from build123d import *

# Parameters (mm, degrees)
BOSS_EXTRUDE1_DEPTH = 12
SKETCH3_R           = 11
CUT_EXTRUDE1_DEPTH  = 12
FILLET1_R           = 15
FILLET2_R           = 15
FILLET3_R           = 2
FILLET4_R           = 2
SKETCH4_R           = 2.5
CUT_EXTRUDE2_DEPTH  = 12
FILLET5_R           = 2
FILLET6_R           = 2
FILLET7_R           = 2
FILLET8_R           = 2


with BuildPart() as part:
    # Sketch2 → Boss-Extrude1 (new body)
    with BuildSketch(Plane(origin=(0, 0, 0), x_dir=(1, 0, 0), z_dir=(0, 1, 0))):
        Polygon((0, 0), (55, 0), (55, 5), (43, 5), (43, 30), (12, 30), (12, 5), (0, 5), align=None)
    extrude(amount=BOSS_EXTRUDE1_DEPTH)

    # Sketch3 → Cut-Extrude1 (cut)
    with BuildSketch(Plane.XZ):
        with Locations(Location((27.5, -17.5, 0), (0, 0, 270))):
            Circle(SKETCH3_R)
    extrude(amount=-CUT_EXTRUDE1_DEPTH, mode=Mode.SUBTRACT)

    # Fillet1
    fillet1_edges = [part.edges().sort_by_distance(p)[0] for p in [
        (43, 6, -30),
    ]]
    fillet(fillet1_edges, radius=FILLET1_R)

    # Fillet2
    fillet2_edges = [part.edges().sort_by_distance(p)[0] for p in [
        (12, 6, -30),
    ]]
    fillet(fillet2_edges, radius=FILLET2_R)

    # Fillet3
    fillet3_edges = [part.edges().sort_by_distance(p)[0] for p in [
        (12, 6, -5),
    ]]
    fillet(fillet3_edges, radius=FILLET3_R)

    # Fillet4
    fillet4_edges = [part.edges().sort_by_distance(p)[0] for p in [
        (43, 6, -5),
    ]]
    fillet(fillet4_edges, radius=FILLET4_R)

    # Sketch4 → Cut-Extrude2 (cut)
    with BuildSketch(Plane.XY):
        with Locations((48.5, 6.034122725)):
            Circle(SKETCH4_R)
        with Locations((6.5, 6.034122725)):
            Circle(SKETCH4_R)
    extrude(amount=-CUT_EXTRUDE2_DEPTH, mode=Mode.SUBTRACT)

    # Fillet5
    fillet5_edges = [part.edges().sort_by_distance(p)[0] for p in [
        (55, 0, -2.5),
    ]]
    fillet(fillet5_edges, radius=FILLET5_R)

    # Fillet6
    fillet6_edges = [part.edges().sort_by_distance(p)[0] for p in [
        (55, 12, -2.5),
    ]]
    fillet(fillet6_edges, radius=FILLET6_R)

    # Fillet7
    fillet7_edges = [part.edges().sort_by_distance(p)[0] for p in [
        (0, 12, -2.5),
    ]]
    fillet(fillet7_edges, radius=FILLET7_R)

    # Fillet8
    fillet8_edges = [part.edges().sort_by_distance(p)[0] for p in [
        (0, 0, -2.5),
    ]]
    fillet(fillet8_edges, radius=FILLET8_R)


solid = part.part
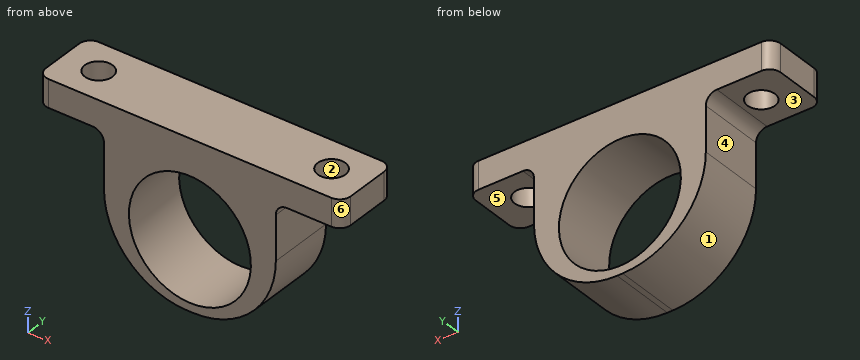
Could you check a few things on this model? Use its own coordinates, in mm. Face numbers are marked on the shaded views. A direction names the side the tool comes from. Give positions to 0.01 mm unless a question says otherwise; leave off trailing zeros. Write each loop counter-clockwise with the first axis right and the second up, starting at its lowest first coordinate (ties: lowest second). Pieces come first, ordered by that corner, then holes. Notation, with made-up numbers: (-4.5, 66.5) -> (6.5, 66.5) arc R17 cw to (6.5, 80.5) -> close; hole circle Ø8 at (1.25, 6). An arc over 180 degrees is marked (long way). Answer as CSV lines item,"result". Start each with the question number.
(1) Please list where these lines run through material, in increasing order: line 1 (Y direction, x = 48.5, z = -2.25); line 2 (X direction, y = 5.25, z = -22.5); line 3 (X direction, y = 7.75, z = -8).
(2) If we section it at A-A, the plane y = 5.5: Write out the boundary of the cut face in (x, z).
(3) Which directions (+Z, -Z, +X, -X, +Y, -Y) give clear straight access to the entire face, cutting with the end or side of a thin tool? Please do the marked faces 4, 5 and 6.
(4) I'm going to push flat-ended pins straight in: pin 1 Ø1 at (x, y) = (15, 10.5) entering from -Z; pin 2 Ø2 at (x, z) = (34, -22.5) entering from +Y; pin 3 Ø6.5 at (x, y) = (48.5, 6.03) entering from +Z; pin 4 Ø3 at (x, y) = (5.5, 7.5) entering from -Z. Where does each tip first touch, or does it pass through?
(5) If we mould it in two halves opening along X, with no side actions, what happens to the marked faces 1, 2 and 3? For each: +X half, -X half, draft (parallel to the pull), parting line (faces both ways), or undercut.
(6) If we section it at C-C, the plane z = -21: Write out the boundary of the cut face in (x, y), and give its area (3 significant figures).
(7) If we section it at B-B, the plane x = 48.5: Write out the boundary of the cut face in (y, z), and give its area (3 significant figures).
Answer list:
1,line 1,"0 to 3.53, 8.53 to 12"
1,line 2,"14.01 to 17.7, 37.3 to 40.99"
1,line 3,"12 to 21.95, 33.05 to 43"
2,outline,"(0, -5) -> (4.06, -5) -> (4.06, 0) -> (0, 0) -> close; (8.94, -5) -> (10, -5) arc R2 cw to (12, -7) -> (12, -15) arc R15 ccw to (27, -30) -> (28, -30) arc R15 ccw to (43, -15) -> (43, -7) arc R2 cw to (45, -5) -> (46.06, -5) -> (46.06, 0) -> (8.94, 0) -> close; (50.94, -5) -> (55, -5) -> (55, 0) -> (50.94, 0) -> close; hole circle Ø22 at (27.5, -17.5)"
3,face 4,"-Z, -X, +Y, -Y"
3,face 5,"-Z, +X, +Y, -Y"
3,face 6,"+Z, -Z, +X, -Y"
4,pin 1,"z = -24.63"
4,pin 2,"through"
4,pin 3,"z = 0"
4,pin 4,"z = -5"
5,face 1,"-X half"
5,face 2,"undercut"
5,face 3,"draft"
6,outline,"(13.25, 0) -> (17.07, 0) -> (17.07, 12) -> (13.25, 12) -> close; (37.93, 0) -> (41.75, 0) -> (41.75, 12) -> (37.93, 12) -> close"
6,area,"91.7 mm^2"
7,outline,"(0, -5) -> (3.53, -5) -> (3.53, 0) -> (0, 0) -> close; (8.53, -5) -> (12, -5) -> (12, 0) -> (8.53, 0) -> close"
7,area,"35.0 mm^2"
